```python
from build123d import *

# Parameters (mm, degrees)
SKETCH_1_W          = 125
SKETCH_1_H          = 80
EXTRUDE_1_DEPTH     = 40
SKETCH_2_W          = 120.2
SKETCH_2_H          = 75.2
CUT_EXTRUDE_1_DEPTH = 37.6
FILLET_1_R          = 1
FILLET_2_R          = 1
SKETCH_7_W          = 121.6
SKETCH_7_H          = 76.6
CUT_EXTRUDE_4_DEPTH = 2


with BuildPart() as part:
    # Эскиз1 → Бобышка-Вытянуть1 (new body)
    with BuildSketch(Plane.XY):
        Rectangle(SKETCH_1_W, SKETCH_1_H)
    extrude(amount=EXTRUDE_1_DEPTH)

    # Эскиз2 → Вырез-Вытянуть1 (cut)
    with BuildSketch(Plane.XY.offset(40)):
        Rectangle(SKETCH_2_W, SKETCH_2_H)
    extrude(amount=-CUT_EXTRUDE_1_DEPTH, mode=Mode.SUBTRACT)

    # Скругление1
    fillet_1_edges = [part.edges().sort_by_distance(p)[0] for p in [
        (0, -40, 0),
        (-62.5, 0, 0),
        (0, 40, 0),
        (62.5, 0, 0),
        (62.5, -40, 20),
        (-62.5, -40, 20),
        (-62.5, 40, 20),
        (62.5, 40, 20),
    ]]
    fillet(fillet_1_edges, radius=FILLET_1_R)

    # Скругление2
    fillet_2_edges = [part.edges().sort_by_distance(p)[0] for p in [
        (60.1, 0, 2.4),
        (60.1, 37.6, 21.2),
        (0, -37.6, 2.4),
        (60.1, -37.6, 21.2),
        (-60.1, 0, 2.4),
        (-60.1, -37.6, 21.2),
        (0, 37.6, 2.4),
        (-60.1, 37.6, 21.2),
    ]]
    fillet(fillet_2_edges, radius=FILLET_2_R)

    # Эскиз7 → Вырез-Вытянуть4 (cut)
    with BuildSketch(Plane.XY.offset(40)):
        with BuildLine():
            ThreePointArc((-62.5, -39), (-62.207106781, -39.707106781), (-61.5, -40))
            Line((-61.5, -40), (61.5, -40))
            ThreePointArc((61.5, -40), (62.207106781, -39.707106781), (62.5, -39))
            Line((62.5, -39), (62.5, 39))
            ThreePointArc((62.5, 39), (62.207106781, 39.707106781), (61.5, 40))
            Line((61.5, 40), (-61.5, 40))
            ThreePointArc((-61.5, 40), (-62.207106781, 39.707106781), (-62.5, 39))
            Line((-62.5, 39), (-62.5, -39))
        make_face()
        Rectangle(SKETCH_7_W, SKETCH_7_H, mode=Mode.SUBTRACT)
    extrude(amount=-CUT_EXTRUDE_4_DEPTH, mode=Mode.SUBTRACT)


solid = part.part
```
Part model, mm, in its own coordinate system. A direction names the side the tool comes from. Coordinates: 2 decimals unless noted, no trailing zeros. Order: outer loops, then holes, each group sorted by start corner. A loop starts at its lowest first (then second) coordinate and runs counter-clockwise, first axis right, second up. Notation, with made-up numbers: (79, -5.5) -> (94, -5.5) arc R26 ccw to (94, 25.5) -> close; hole circle Ø6 at (-7, 30). An arc over 180 degrees is marked (long way). Put each result on its own line as item: value. Start each with the question number.
(1) Band-saw the part on C-C (y = 27). Give the cut face in (x, z).
(2) Mould opens along X. For faces 1 (the face through (-1, 37.6, 22)), 2 (the face through (-1, -40, 19)), 3 (the face through (-62.5, -1, 19)), 4 (the face through (-1, -37.6, 22)) say: pulls with the +X half, pulls with the -X half, needs draft (parallel to the pull), parting line crosses it, or undercut.
(3) Pin check, flat tips, straight feed: pin 1 Ø2 at (x, z) = (22.5, 39.5) entering from -Y; pin 2 Ø0.6 at (y, z) = (-14, 38.5) entering from +X; pin 3 Ø22 at (x, y) = (-4, 15) entering from +Z. Stop position of each tip, or through.
(4) Band-saw the part on B-B (x = -37.5). Give the cut face in (y, z).
(5) Probe line 1 along X through (y, z) = (-33, 34); line 2 along Y through (x, z) = (43, 16); line 3 along Z through (x, y) = (54, -3). List the from-to ranges inside material, lowest first. Write a range as [from, to].
(6) Band-saw the part on A-A (z = 7). Give the cut face in (x, y).
(7) Which spindle directions (+Z, -Z, +X, -X, +Y, -Y) get a long thin tool onto all of the face, cutting with end or side? Do faces 5 (the face through (-1, 40, 19)), 6 (the face through (-60.1, -1, 22)). Say none if no direction does.
Determined:
1. outline: (-62.5, 1) arc R1 ccw to (-61.5, 0) -> (61.5, 0) arc R1 ccw to (62.5, 1) -> (62.5, 38) -> (60.8, 38) -> (60.8, 40) -> (60.1, 40) -> (60.1, 3.4) arc R1 cw to (59.1, 2.4) -> (-59.1, 2.4) arc R1 cw to (-60.1, 3.4) -> (-60.1, 40) -> (-60.8, 40) -> (-60.8, 38) -> (-62.5, 38) -> close
2. face 1: undercut
2. face 2: needs draft
2. face 3: pulls with the -X half
2. face 4: undercut
3. pin 1: stops at y = -38.3
3. pin 2: stops at x = 60.8
3. pin 3: stops at z = 2.4
4. outline: (-40, 1) arc R1 ccw to (-39, 0) -> (39, 0) arc R1 ccw to (40, 1) -> (40, 38) -> (38.3, 38) -> (38.3, 40) -> (37.6, 40) -> (37.6, 3.4) arc R1 cw to (36.6, 2.4) -> (-36.6, 2.4) arc R1 cw to (-37.6, 3.4) -> (-37.6, 40) -> (-38.3, 40) -> (-38.3, 38) -> (-40, 38) -> close
5. line 1: x = [-62.5, -60.1], [60.1, 62.5]
5. line 2: y = [-40, -37.6], [37.6, 40]
5. line 3: z = [0, 2.4]
6. outline: (-62.5, -39) arc R1 ccw to (-61.5, -40) -> (61.5, -40) arc R1 ccw to (62.5, -39) -> (62.5, 39) arc R1 ccw to (61.5, 40) -> (-61.5, 40) arc R1 ccw to (-62.5, 39) -> close; hole (-60.1, -36.6) arc R1 ccw to (-59.1, -37.6) -> (59.1, -37.6) arc R1 ccw to (60.1, -36.6) -> (60.1, 36.6) arc R1 ccw to (59.1, 37.6) -> (-59.1, 37.6) arc R1 ccw to (-60.1, 36.6) -> close
7. face 5: +Z, -Z, +X, -X, +Y
7. face 6: +Z
